```python
from build123d import *

# Parameters (mm, degrees)
F0_W     = 98.122775
F0_H     = 53.054758
F1_DEPTH = 56.388
F2_W     = 72.451114
F2_H     = 39.933689
F3_DEPTH = 56.389
F4_R     = 6.804049
F5_DEPTH = 106.39576
F7_DEPTH = 101.6


with BuildPart() as f1:
    # F0 (on Top) → F1 (new body)
    with BuildSketch(Plane.XY):
        with Locations((57.333372, -39.505832)):
            Rectangle(F0_W, F0_H)
    extrude(amount=F1_DEPTH)

    # F2 (on Top) → F3 (cut, through all)
    with BuildSketch(Plane.XY):
        with Locations((57.598237, -39.791069)):
            Rectangle(F2_W, F2_H)
    extrude(amount=F3_DEPTH, mode=Mode.SUBTRACT)

    # F4 (on Right) → F5 (cut, through all)
    with BuildSketch(Plane.YZ):
        with Locations((-40.218931, 29.807648)):
            Circle(F4_R)
    extrude(amount=F5_DEPTH, mode=Mode.SUBTRACT)

    # F6 (on Front) → F7 (cut)
    with BuildSketch(Plane.XZ):
        Polygon((84.981345, 64.892247), (40.198553, 62.610321), (29.074172, 62.610321), (29.074172, 32.089572), (84.981345, 32.089572), align=None)
    extrude(amount=F7_DEPTH, mode=Mode.SUBTRACT)


solid = f1.part
```
The model under review builds one solid part; all positions refer to its coordinate system, in mm. A direction names the side the tool comes from. Give positions to 0.01 mm unless a question says otherwise; leave off trailing zeros. Loops run counter-clockwise (first coordinate to the right, second up) from the corner with the lowest first, then second, coordinate; pieces in that order, holes last. Notation, with made-up numbers: (-19, 80) - (11, 80) arc R19 cw to (11, 85) - close; hole circle Ø4 at (72.5, 89). An arc over 180 degrees is marked (long way). Answer as a JSON object with one key per item and string values.
Q1. Add section C-C on z = 17. State the section outline as (x, y) points.
Worked out:
{"outline": "(8.27, -66.03) - (106.39, -66.03) - (106.39, -12.98) - (8.27, -12.98) - close; hole (21.37, -59.76) - (93.82, -59.76) - (93.82, -19.82) - (21.37, -19.82) - close"}
Q2. Add section A-A on x = 50.5. State the section outline as (y, z) points.
Worked out:
{"outline": "(-66.03, 0) - (-59.76, 0) - (-59.76, 32.09) - (-66.03, 32.09) - close; (-19.82, 0) - (-12.98, 0) - (-12.98, 32.09) - (-19.82, 32.09) - close"}
Q3. To check wall thickness, follow line 1 along Y through (x, z) = (71.5, 24.5); line 2 along X through (y, z) = (-54.5, 37); line 3 along Y through (x, z) = (99.5, 30). State the ranges of each line that lie inside material, in increasing order.
Worked out:
{"line 1": "y = -66.03 to -59.76, -19.82 to -12.98", "line 2": "x = 8.27 to 21.37, 93.82 to 106.39", "line 3": "y = -66.03 to -47.02, -33.42 to -12.98"}
Q4. For faces 1 (the flat face through (106.395, -40, 22)), 2 (the flat face through (57, -59.758, 22)), 3 (the flat face through (57, -16, 32.09)), list the 3-axis set-ups (+Z, -Z, +X, -X, +Y, -Y) from which the entire face can be reached by the end or side of a thin tool; tool diameter is ignored.
Worked out:
{"face 1": "+Z, -Z, +X, +Y, -Y", "face 2": "+Z, -Z", "face 3": "+Z, +Y, -Y"}
Q5. Insertion check: pin 1 (7.5 mm diameter, centred on x = 48.5, y = -16.5, fed in from +Z); pin 2 (15.5 mm diameter, centred on y = -40.22, z = 29.81, fed in from -X). Each pin has a flat end and moves straight along its axis. Give the tip position at first contact, or say it passes through.
Worked out:
{"pin 1": "stops at z = 32.09", "pin 2": "stops at x = 8.27"}
Q6. Mouldability with a two-part tool opening along X and no side actions: class faces 4 (the flat face through (57, -66.033, 22)), 5 (the flat face through (8.272, -40, 22)), 6 (the flat face through (93.824, -40, 22)) as +X half, -X half, draft (parallel to the pull), parting line (faces both ways), or undercut.
Worked out:
{"face 4": "draft", "face 5": "-X half", "face 6": "undercut"}
Q7. Add section B-B on y = -22. State the section outline as (x, z) points.
Worked out:
{"outline": "(8.27, 0) - (21.37, 0) - (21.37, 56.39) - (8.27, 56.39) - close; (93.82, 0) - (106.39, 0) - (106.39, 56.39) - (93.82, 56.39) - close"}
Q8. Add section D-D on z = 48. State the section outline as (x, y) points, plus the area to 3 significant figures.
Worked out:
{"outline": "(8.27, -66.03) - (29.07, -66.03) - (29.07, -59.76) - (21.37, -59.76) - (21.37, -19.82) - (29.07, -19.82) - (29.07, -12.98) - (8.27, -12.98) - close; (84.98, -66.03) - (106.39, -66.03) - (106.39, -12.98) - (84.98, -12.98) - (84.98, -19.82) - (93.82, -19.82) - (93.82, -59.76) - (84.98, -59.76) - close", "area": "1,580 mm^2"}
